Can you work these out from the model? Positions are in its coordinate system, mm. A direction names the side the tool comes from. Round coordinates to 2 decimals unless told otherwise and drop trailing zeros. Write each loop counter-clockwise with the first axis right and the second up, starting at its lowest first coordinate (ties: lowest second). Pieces come first, ordered by that corner, then holes. Notation, with made-up numbers: M 35,-26.75 L 54,-26.75 A20 ccw 54,10.25 Z; hole C 52.5,80.25 d8. An arc over 180 degrees is marked long. Answer as a JSON object with one key per item and string values. Group by question number.
1) On a 3-axis mill with a long thin cutter (end or side, diameter ignored), from which of +Z, -Z, +X, -X, +Y, -Y can I reach the whole of each face in a straight line? I mean faces 1 (the flat face through (-153.306, 113.907, 2.958)), 2 (the flat face through (-217, 118.624, 7)), 3 (the flat face through (-215, 102.124, 10)), 4 (the cylindrical face through (-214.025, 141.454, 6.354)). Say none if no direction works.
2) If we mould it in two halves opening along Z, with no side actions, what happens to faces 5 (the flat face through (-73.49, 117.81, 2.96)), 6 (the flat face through (-217, 115, 21.1)), 7 (the flat face through (-124, 89, 6))? For each: +Z half, -Z half, draft (parallel to the pull), parting line (faces both ways), or undercut.
3) Please list where these lines run through material, in increasing order: L1, parallel to X at y = 134.5, z = 4.75; L2, parallel to Z at x = -206.5, y = 108; L3, parallel to X at y = 119.5, z = 2.25. Write a range as [from, to].
4) Suppose I cut it at C-C, the plane z = 15. Write out the boundary of the cut face in (x, y).
5) Suppose I cut it at B-B, the plane y = 116. Write out the boundary of the cut face in (x, z).
6) Suppose I cut it at A-A, the plane y = 98. Write out the boundary of the cut face in (x, z).
7) I'm going to push flat-ended pins straight in: pin 1 Ø1 at (y, z) = (145.5, 4) entering from +X; pin 2 Ø6.5 at (x, z) = (-30.5, 1.5) entering from +Y; pin 3 Ø1.2 at (x, z) = (-217, 6.5) entering from -Y; pin 4 Ø0.9 at (x, z) = (-211.77, 3) entering from -Y. Where does each tip first touch, or does it pass through?
from build123d import *

# Parameters (mm, degrees)
BOSS_EXTRUDE1_DEPTH = 6
SKETCH2_R           = 1.1
CUT_EXTRUDE1_DEPTH  = 6
SKETCH3_R           = 0.75
CUT_EXTRUDE2_DEPTH  = 6
SKETCH4_R           = 0.75
CUT_EXTRUDE3_DEPTH  = 6
SKETCH5_R           = 0.75
CUT_EXTRUDE4_DEPTH  = 6
SKETCH6_R           = 0.75
CUT_EXTRUDE5_DEPTH  = 6
SKETCH7_R           = 0.75
CUT_EXTRUDE6_DEPTH  = 6
SKETCH8_R           = 0.75
CUT_EXTRUDE7_DEPTH  = 6
SKETCH9_R           = 0.75
CUT_EXTRUDE8_DEPTH  = 6
SKETCH12_W          = 20
SKETCH12_H          = 45
BOSS_EXTRUDE5_DEPTH = 4
FILLET4_R           = 4
SKETCH13_W          = 19
SKETCH13_H          = 45
BOSS_EXTRUDE6_DEPTH = 2
FILLET5_R           = 3
SKETCH14_W          = 4.2
SKETCH14_H          = 7
CUT_EXTRUDE10_DEPTH = 12


with BuildPart() as part:
    # Sketch1 → Boss-Extrude1 (new body)
    with BuildSketch(Plane.XY):
        Polygon((-23.705812739, 144.922992632), (-23.705812739, 142.922992632), (-61.705812739, 142.922992632), (-79.093908962, 85.497788151), (-145.066881196, 85.497788151), (-161.778348211, 143.123536478), (-214.773543294, 143.123536478), (-214.773543294, 102.123536478), (-218.773543294, 102.123536478), (-218.773543294, 147.123536478), (-158.773543294, 147.123536478), (-142.062076279, 89.497788151), (-82.062076279, 89.497788151), (-64.673980056, 146.922992632), (-43.605812739, 146.922992632), (-43.605812739, 144.922992632), align=None)
    extrude(amount=BOSS_EXTRUDE1_DEPTH)

    # Sketch2 → Cut-Extrude1 (cut)
    with BuildSketch(Plane(origin=(0, 144.922992632, 0), x_dir=(1, 0, 0), z_dir=(0, 1, 0))):
        with Locations(Location((-28.605812739, -3, 0), (0, 0, 270))):
            Circle(SKETCH2_R)
        with Locations(Location((-40.605812739, -3, 0), (0, 0, 270))):
            Circle(SKETCH2_R)
    extrude(amount=-CUT_EXTRUDE1_DEPTH, mode=Mode.SUBTRACT)

    # Sketch3 → Cut-Extrude2 (cut)
    with BuildSketch(Plane(origin=(0, 144.922992632, 0), x_dir=(1, 0, 0), z_dir=(0, 1, 0))):
        with Locations(Location((-34.605812739, -3, 0), (0, 0, 270))):
            Circle(SKETCH3_R)
    extrude(amount=-CUT_EXTRUDE2_DEPTH, mode=Mode.SUBTRACT)

    # Sketch4 → Cut-Extrude3 (cut)
    with BuildSketch(Plane(origin=(0, 146.922992632, 0), x_dir=(1, 0, 0), z_dir=(0, 1, 0))):
        with Locations(Location((-59.673980056, -3, 0), (0, 0, 270))):
            Circle(SKETCH4_R)
        with Locations(Location((-49.673980056, -3, 0), (0, 0, 270))):
            Circle(SKETCH4_R)
    extrude(amount=-CUT_EXTRUDE3_DEPTH, mode=Mode.SUBTRACT)

    # Sketch5 → Cut-Extrude4 (cut)
    with BuildSketch(Plane(origin=(-99.993673707, 30.277639163, 0), x_dir=(0, 0, 1), z_dir=(-0.957086741355951, 0.28980160372338726, 0))):
        with Locations(Location((3, 116.875425109, 0), (0, 0, 270))):
            Circle(SKETCH5_R)
        with Locations(Location((3, 106.875425109, 0), (0, 0, 270))):
            Circle(SKETCH5_R)
        with Locations(Location((3, 96.875425109, 0), (0, 0, 270))):
            Circle(SKETCH5_R)
        with Locations(Location((3, 86.875425109, 0), (0, 0, 270))):
            Circle(SKETCH5_R)
        with Locations(Location((3, 76.875425109, 0), (0, 0, 270))):
            Circle(SKETCH5_R)
        with Locations(Location((3, 66.875425109, 0), (0, 0, 270))):
            Circle(SKETCH5_R)
    extrude(amount=-CUT_EXTRUDE4_DEPTH, mode=Mode.SUBTRACT)

    # Sketch6 → Cut-Extrude5 (cut)
    with BuildSketch(Plane(origin=(0, 89.497788151, 0), x_dir=(1, 0, 0), z_dir=(0, 1, 0))):
        with Locations(Location((-87.062076279, -3, 0), (0, 0, 270))):
            Circle(SKETCH6_R)
        with Locations(Location((-97.062076279, -3, 0), (0, 0, 270))):
            Circle(SKETCH6_R)
        with Locations(Location((-107.062076279, -3, 0), (0, 0, 270))):
            Circle(SKETCH6_R)
        with Locations(Location((-117.062076279, -3, 0), (0, 0, 270))):
            Circle(SKETCH6_R)
        with Locations(Location((-127.062076279, -3, 0), (0, 0, 270))):
            Circle(SKETCH6_R)
        with Locations(Location((-137.062076279, -3, 0), (0, 0, 270))):
            Circle(SKETCH6_R)
    extrude(amount=-CUT_EXTRUDE5_DEPTH, mode=Mode.SUBTRACT)

    # Sketch7 → Cut-Extrude6 (cut)
    with BuildSketch(Plane(origin=(-107.100560571, -31.059162566, 0), x_dir=(0, 0, -1), z_dir=(0.960429138778729, 0.27852445024584294, 0))):
        with Locations(Location((-3, 180.524045293, 0), (0, 0, 90))):
            Circle(SKETCH7_R)
        with Locations(Location((-3, 170.524045293, 0), (0, 0, 90))):
            Circle(SKETCH7_R)
        with Locations(Location((-3, 160.524045293, 0), (0, 0, 90))):
            Circle(SKETCH7_R)
        with Locations(Location((-3, 150.524045293, 0), (0, 0, 90))):
            Circle(SKETCH7_R)
        with Locations(Location((-3, 140.524045293, 0), (0, 0, 90))):
            Circle(SKETCH7_R)
        with Locations(Location((-3, 130.524045293, 0), (0, 0, 90))):
            Circle(SKETCH7_R)
    extrude(amount=-CUT_EXTRUDE6_DEPTH, mode=Mode.SUBTRACT)

    # Sketch8 → Cut-Extrude7 (cut)
    with BuildSketch(Plane(origin=(0, 147.123536478, 0), x_dir=(1, 0, 0), z_dir=(0, 1, 0))):
        with Locations(Location((-211.773543294, -3, 0), (0, 0, 270))):
            Circle(SKETCH8_R)
        with Locations(Location((-201.773543294, -3, 0), (0, 0, 270))):
            Circle(SKETCH8_R)
        with Locations(Location((-191.773543294, -3, 0), (0, 0, 270))):
            Circle(SKETCH8_R)
        with Locations(Location((-181.773543294, -3, 0), (0, 0, 270))):
            Circle(SKETCH8_R)
        with Locations(Location((-171.773543294, -3, 0), (0, 0, 270))):
            Circle(SKETCH8_R)
    extrude(amount=-CUT_EXTRUDE7_DEPTH, mode=Mode.SUBTRACT)

    # Sketch9 → Cut-Extrude8 (cut)
    with BuildSketch(Plane(origin=(0, 147.123536478, 0), x_dir=(1, 0, 0), z_dir=(0, 1, 0))):
        with Locations(Location((-163.773543294, -3, 0), (0, 0, 270))):
            Circle(SKETCH9_R)
    extrude(amount=-CUT_EXTRUDE8_DEPTH, mode=Mode.SUBTRACT)

    # Sketch12 → Boss-Extrude5 (add)
    with BuildSketch(Plane.ZY.offset(218.773543294)):
        with Locations((16, 124.623536478)):
            Rectangle(SKETCH12_W, SKETCH12_H)
    extrude(amount=-BOSS_EXTRUDE5_DEPTH)

    # Fillet4
    # the kernel refuses this fillet: 4 mm, written as the material it adds along each edge
    with BuildSketch(Plane(origin=(-214.773543294, 143.123536478, 6), x_dir=(1, 0, 0), z_dir=(0, 1, 0))) as fillet4_piece_1:
        with BuildLine():
            CenterArc((FILLET4_R, -FILLET4_R), FILLET4_R, 90, 90)
            Line((0, -FILLET4_R), (0, 0))
            Line((0, 0), (FILLET4_R, 0))
        make_face()
    extrude(amount=4)
    with BuildSketch(Plane(origin=(-214.773543294, 143.123536478, 0), x_dir=(1, 0, 0), z_dir=(0, 0, 1))) as fillet4_piece_2_section:
        with BuildLine():
            CenterArc((FILLET4_R, -FILLET4_R), FILLET4_R, 90, 90)
            Line((0, -FILLET4_R), (0, 0))
            Line((0, 0), (FILLET4_R, 0))
        make_face()
    fillet4_piece_2 = extrude(amount=6, mode=Mode.PRIVATE)
    fillet4_piece_2 = fillet4_piece_2 - Plane(origin=(-211.773543294, 142.203820796, 3), x_dir=(0, 0, 1), z_dir=(0, 1, 0)) * Cylinder(0.75, 28, mode=Mode.PRIVATE)
    add(fillet4_piece_2)
    with BuildSketch(Plane(origin=(-214.773543294, 133.123536478, 6), x_dir=(1, 0, 0), z_dir=(0, 1, 0))) as fillet4_piece_3a_section:
        with BuildLine():
            CenterArc((FILLET4_R, -FILLET4_R), FILLET4_R, 90, 90)
            Line((0, -FILLET4_R), (0, 0))
            Line((0, 0), (FILLET4_R, 0))
        make_face()
    fillet4_piece_3a = extrude(amount=14, mode=Mode.PRIVATE)
    fillet4_piece_3a = split(fillet4_piece_3a, bisect_by=Plane(origin=(-213.867962837, 143.123536478, 6.905580457), z_dir=(0, -1, 0)), keep=Keep.TOP, mode=Mode.PRIVATE)
    with BuildSketch(Plane(origin=(-214.773543294, 143.123536478, 0), x_dir=(1, 0, 0), z_dir=(0, 0, 1))) as fillet4_piece_3b_section:
        with BuildLine():
            CenterArc((FILLET4_R, -FILLET4_R), FILLET4_R, 90, 90)
            Line((0, -FILLET4_R), (0, 0))
            Line((0, 0), (FILLET4_R, 0))
        make_face()
    fillet4_piece_3b = extrude(amount=16, mode=Mode.PRIVATE)
    fillet4_piece_3b = split(fillet4_piece_3b, bisect_by=Plane(origin=(-213.867962837, 142.217956021, 6), z_dir=(0, 0, 1)), keep=Keep.TOP, mode=Mode.PRIVATE)
    fillet4_piece_3 = fillet4_piece_3a & fillet4_piece_3b
    add(fillet4_piece_3)

    # Sketch13 → Boss-Extrude6 (add)
    with BuildSketch(Plane(origin=(0, 0, 0), x_dir=(-1, 0, 0), z_dir=(0, 0, -1))):
        with Locations((209.273543294, 124.623536478)):
            Rectangle(SKETCH13_W, SKETCH13_H)
    extrude(amount=-BOSS_EXTRUDE6_DEPTH)

    # Fillet5
    # the kernel refuses this fillet: 3 mm, written as the material it adds along each edge
    with BuildSketch(Plane(origin=(-210.773543294, 139.123536478, 2), x_dir=(-1, 0, 0), z_dir=(0, -1, 0))) as fillet5_piece_1_section:
        with BuildLine():
            CenterArc((4 - FILLET5_R, -FILLET5_R), FILLET5_R, 0, 90)
            Line((4, -FILLET5_R), (4, 0))
            Line((4, 0), (4 - FILLET5_R, 0))
        make_face()
    fillet5_piece_1 = revolve(axis=Axis((-210.773543294, 139.123536478, 2), (0, 0, -1)), revolution_arc=90, mode=Mode.PRIVATE)
    fillet5_piece_1 = fillet5_piece_1 - Plane(origin=(-211.773543294, 141.130848213, 3), x_dir=(0, 0, 1), z_dir=(0, 1, 0)) * Cylinder(0.75, 16, mode=Mode.PRIVATE)
    add(fillet5_piece_1)
    with BuildSketch(Plane(origin=(-199.773543294, 143.123536478, 0), x_dir=(0, -1, 0), z_dir=(0, 0, 1))) as fillet5_piece_2:
        with BuildLine():
            CenterArc((FILLET5_R, FILLET5_R), FILLET5_R, 180, 90)
            Line((0, FILLET5_R), (0, 0))
            Line((0, 0), (FILLET5_R, 0))
        make_face()
    extrude(amount=2)
    with BuildSketch(Plane(origin=(-214.773543294, 102.123536478, 2), x_dir=(0, 0, 1), z_dir=(0, 1, 0))) as fillet5_piece_3:
        with BuildLine():
            CenterArc((FILLET5_R, FILLET5_R), FILLET5_R, 180, 90)
            Line((0, FILLET5_R), (0, 0))
            Line((0, 0), (FILLET5_R, 0))
        make_face()
    extrude(amount=37)
    with BuildSketch(Plane(origin=(-210.773543294, 143.123536478, 2), x_dir=(0, 0, 1), z_dir=(1, 0, 0))) as fillet5_piece_4_section:
        with BuildLine():
            CenterArc((FILLET5_R, FILLET5_R), FILLET5_R, 180, 90)
            Line((0, FILLET5_R), (0, 0))
            Line((0, 0), (FILLET5_R, 0))
        make_face()
    fillet5_piece_4 = extrude(amount=11, mode=Mode.PRIVATE)
    fillet5_piece_4 = fillet5_piece_4 - Plane(origin=(-201.773543294, 142.429647528, 3), x_dir=(0, 0, 1), z_dir=(0, 1, 0)) * Cylinder(0.75, 35, mode=Mode.PRIVATE)
    add(fillet5_piece_4)
    with BuildSketch(Plane(origin=(-199.773543294, 143.123536478, 0), x_dir=(0, -1, 0), z_dir=(0, 0, 1))) as fillet5_piece_5a_section:
        with BuildLine():
            CenterArc((FILLET5_R, FILLET5_R), FILLET5_R, 180, 90)
            Line((0, FILLET5_R), (0, 0))
            Line((0, 0), (FILLET5_R, 0))
        make_face()
    fillet5_piece_5a = extrude(amount=9.5, mode=Mode.PRIVATE)
    fillet5_piece_5a = split(fillet5_piece_5a, bisect_by=Plane(origin=(-199.094357951, 142.444351135, 2), z_dir=(0, 0, 1)), keep=Keep.TOP, mode=Mode.PRIVATE)
    fillet5_piece_5a = split(fillet5_piece_5a, bisect_by=Plane(origin=(-199.094357951, 142.444351135, 6), z_dir=(0, 0, -1)), keep=Keep.TOP, mode=Mode.PRIVATE)
    with BuildSketch(Plane(origin=(-210.773543294, 143.123536478, 2), x_dir=(0, 0, 1), z_dir=(1, 0, 0))) as fillet5_piece_5b_section:
        with BuildLine():
            CenterArc((FILLET5_R, FILLET5_R), FILLET5_R, 180, 90)
            Line((0, FILLET5_R), (0, 0))
            Line((0, 0), (FILLET5_R, 0))
        make_face()
    fillet5_piece_5b = extrude(amount=18.5, mode=Mode.PRIVATE)
    fillet5_piece_5b = split(fillet5_piece_5b, bisect_by=Plane(origin=(-199.773543294, 142.441638418, 2.676766497), z_dir=(1, 0, 0)), keep=Keep.TOP, mode=Mode.PRIVATE)
    fillet5_piece_5b = fillet5_piece_5b - Plane(origin=(-191.773543294, 142.441638418, 3), x_dir=(0, 0, 1), z_dir=(0, 1, 0)) * Cylinder(0.75, 50, mode=Mode.PRIVATE)
    fillet5_piece_5 = fillet5_piece_5a & fillet5_piece_5b
    add(fillet5_piece_5)

    # Sketch14 → Cut-Extrude10 (cut)
    with BuildSketch(Plane.ZY.offset(218.773543294)):
        with Locations((7, 115.123536478)):
            Rectangle(SKETCH14_W, SKETCH14_H)
        with Locations((19, 115.123536478)):
            Rectangle(SKETCH14_W, SKETCH14_H)
    extrude(amount=-CUT_EXTRUDE10_DEPTH, mode=Mode.SUBTRACT)


solid = part.part
Results:
{
 "1": {"face 1": "+Z, -Z, -Y", "face 2": "-X", "face 3": "+Z, -Z, -X, -Y", "face 4": "+Z, -Y"},
 "2": {"face 5": "draft", "face 6": "undercut", "face 7": "+Z half"},
 "3": {"L1": "[-218.77, -214.76], [-159.28, -155.11], [-68.44, -64.26]", "L2": "[0, 2]", "L3": "[-218.77, -212.97], [-154.93, -150.76], [-72.98, -68.8]"},
 "4": {"outline": "M -218.77,102.12 L -214.77,102.12 L -214.77,147.12 L -218.77,147.12 Z"},
 "5": {"outline": "M -218.77,0 L -199.77,0 L -199.77,2 L -211.77,2 A3 cw -214.77,4.9 L -218.77,4.9 Z; M -218.77,9.1 L -214.77,9.1 L -214.77,16.9 L -218.77,16.9 Z; M -218.77,21.1 L -214.77,21.1 L -214.77,26 L -218.77,26 Z; M -153.91,0 L -149.75,0 L -149.75,6 L -153.91,6 Z; M -74.04,0 L -69.86,0 L -69.86,6 L -74.04,6 Z"},
 "6": {"outline": "M -148.69,0 L -144.53,0 L -144.53,6 L -148.69,6 Z; M -79.49,0 L -75.31,0 L -75.31,6 L -79.49,6 Z"},
 "7": {"pin 1": "x = -43.61", "pin 2": "y = 144.92", "pin 3": "y = 102.12", "pin 4": "through"}
}
